For this review, use the dimensioned drawing (mm, ordinates from the lowest corner) and the shaded views. A direction names the side the tool comes from. Give positions to 0.01 mm unless a question says otherwise; leave off trailing zeros. Write each loop counter-clockwise with the first axis right and the second up, starting at its lowest first coordinate (ties: lowest second). Pieces come first, ordered by that corner, then holes.
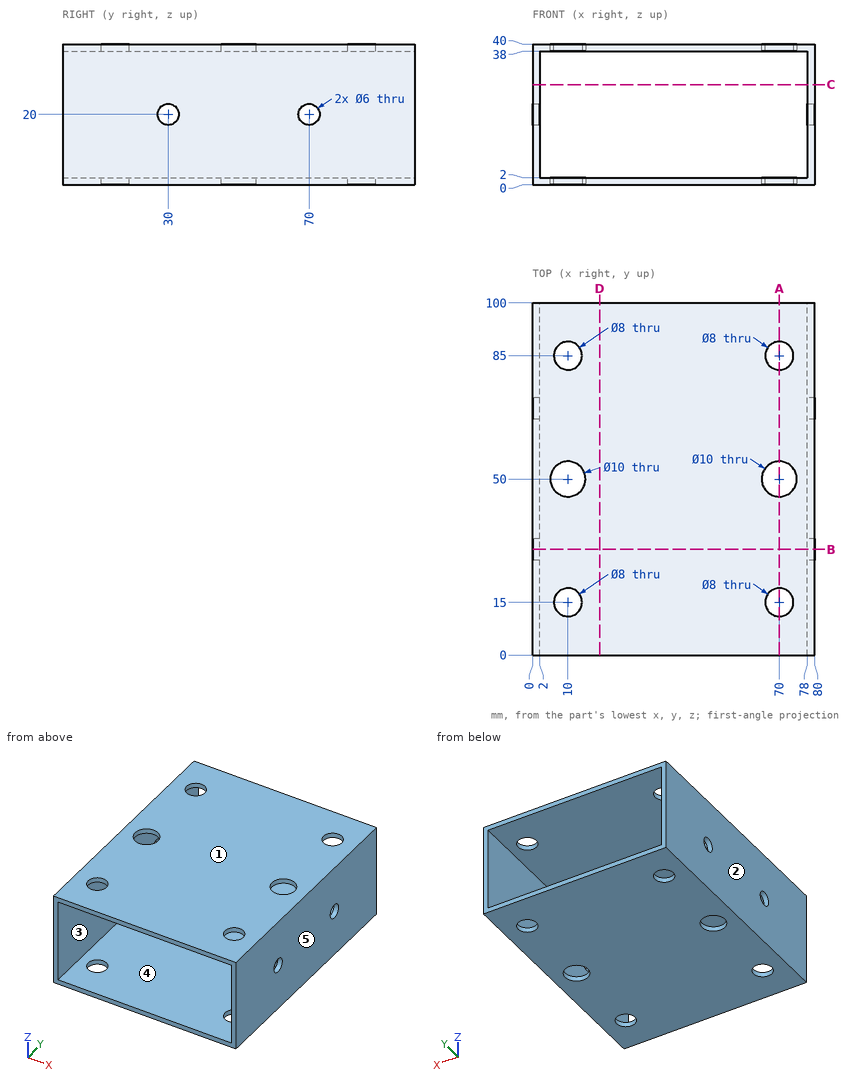
(1) We need section C-C (z = 28.5). Write out the cut boundary in (x, y).
(2) We need section D-D (x = 19). Write out the cut boundary in (y, z), and give its area (3 significant figures).
(3) We need section A-A (x = 70). Count the separate pieces of the cut face and the enclosed holes in it, and give its area (3 significant figures).
(4) The part is to be moulded in two halves that separate along Z. For the marked faces 1, 2 and 3, say which applies: +Z half, -Z half, draft (parallel to the pull), parting line (faces both ways), or undercut.
(5) For L1, parallel to Y at x = 79, z = 20; L2, parallel to X at y = 72, z = 28; L3, parallel to Z at x = 22.5, y = 61, list the stretches that pass through material, from the lowest coordinate up.
(6) Tool access review of the marked faces 4 and 5: name each direction out of +Z, -Z, +X, -X, +Y, -Y from which nothing blocks a thin tool from reaching the whole face with its end or side.
(7) We need section B-B (y = 30). Write out the cut boundary in (x, z), and give its area (3 significant figures).
The answers:
1. outline: (0, 0) - (2, 0) - (2, 100) - (0, 100) - close; (78, 0) - (80, 0) - (80, 100) - (78, 100) - close
2. outline: (0, 0) - (100, 0) - (100, 2) - (0, 2) - close; (0, 38) - (100, 38) - (100, 40) - (0, 40) - close
2. area: 400 mm2
3. separate pieces: 8
3. enclosed holes: 0
3. area: 296 mm2
4. face 1: +Z half
4. face 2: draft
4. face 3: undercut
5. L1: y = 0 to 27, 33 to 67, 73 to 100
5. L2: x = 0 to 2, 78 to 80
5. L3: z = 0 to 2, 38 to 40
6. face 4: +Y, -Y
6. face 5: +Z, -Z, +X, +Y, -Y
7. outline: (0, 0) - (80, 0) - (80, 17) - (78, 17) - (78, 2) - (2, 2) - (2, 17) - (0, 17) - close; (0, 23) - (2, 23) - (2, 38) - (78, 38) - (78, 23) - (80, 23) - (80, 40) - (0, 40) - close
7. area: 440 mm2
